Check sheet for the modelled part. Datum: model origin and axes. Units: mm. Round coordinates to 2 decimals unless told otherwise and drop trailing zeros. Write each loop counter-clockwise with the first axis right and the second up, starting at its lowest first coordinate (ties: lowest second). Pieces come first, ordered by that corner, then holes.
Item 1: Material ranges on line 1 along X through (y, z) = (1.5, -235); line 2 along Z through (x, y) = (219, 1.2); line 3 along Z through (x, y) = (235, 1.9), recorded low to high.
Item 2: Depth check by flat-ended pin: pin 1 (4 mm diameter, centred on x = 57.5, z = -190, fed in from -Y); pin 2 (4.5 mm diameter, centred on x = 15, z = -235, fed in from +Y). Enter the tip coordinate at first touch or a pass-through.
Item 3: Section check B-B, the plane z = -135.5. Record the cut outline in (x, y), plus the area to 3 significant figures.
Item 4: Section check A-A, the plane x = 59. Record the cut outline in (y, z).
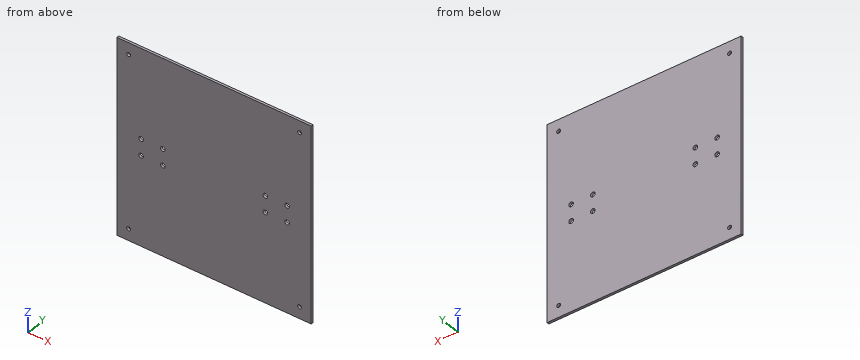
from build123d import *

# Parameters (mm, degrees)
SKETCH1_W           = 250
SKETCH1_H           = 250
BOSS_EXTRUDE1_DEPTH = 3
SKETCH2_R           = 2.5
SKETCH2_R_2         = 3
CUT_EXTRUDE1_DEPTH  = 354.566118286


with BuildPart() as part:
    # Sketch1 → Boss-Extrude1 (new body)
    with BuildSketch(Plane(origin=(0, 0, 0), x_dir=(1, 0, 0), z_dir=(0, 1, 0))):
        with Locations((125, 125)):
            Rectangle(SKETCH1_W, SKETCH1_H)
    extrude(amount=BOSS_EXTRUDE1_DEPTH)

    # Sketch2 → Cut-Extrude1 (cut, through all)
    with BuildSketch(Plane(origin=(0, 3, 0), x_dir=(1, 0, 0), z_dir=(0, 1, 0))):
        with Locations(Location((15, 235, 0), (0, 0, 270))):
            Circle(SKETCH2_R)
        with Locations(Location((235, 235, 0), (0, 0, 270))):
            Circle(SKETCH2_R)
        with Locations(Location((235, 15, 0), (0, 0, 270))):
            Circle(SKETCH2_R)
        with Locations(Location((15, 15, 0), (0, 0, 270))):
            Circle(SKETCH2_R)
        with Locations(Location((31, 135.5, 0), (0, 0, 270))):
            Circle(SKETCH2_R_2)
        with Locations(Location((59, 135.5, 0), (0, 0, 270))):
            Circle(SKETCH2_R_2)
        with Locations(Location((59, 114.5, 0), (0, 0, 270))):
            Circle(SKETCH2_R_2)
        with Locations(Location((31, 114.5, 0), (0, 0, 270))):
            Circle(SKETCH2_R_2)
        with Locations(Location((191, 135.5, 0), (0, 0, 270))):
            Circle(SKETCH2_R_2)
        with Locations(Location((219, 135.5, 0), (0, 0, 270))):
            Circle(SKETCH2_R_2)
        with Locations(Location((219, 114.5, 0), (0, 0, 270))):
            Circle(SKETCH2_R_2)
        with Locations(Location((191, 114.5, 0), (0, 0, 270))):
            Circle(SKETCH2_R_2)
    extrude(amount=-CUT_EXTRUDE1_DEPTH, mode=Mode.SUBTRACT)


solid = part.part
Values found:
1. line 1: x = 0 to 12.5, 17.5 to 232.5, 237.5 to 250
1. line 2: z = -250 to -138.5, -132.5 to -117.5, -111.5 to 0
1. line 3: z = -250 to -237.5, -232.5 to -17.5, -12.5 to 0
2. pin 1: stops at y = 0
2. pin 2: passes through
3. outline: (0, 0) - (28, 0) - (28, 3) - (0, 3) - close; (34, 0) - (56, 0) - (56, 3) - (34, 3) - close; (62, 0) - (188, 0) - (188, 3) - (62, 3) - close; (194, 0) - (216, 0) - (216, 3) - (194, 3) - close; (222, 0) - (250, 0) - (250, 3) - (222, 3) - close
3. area: 678 mm2
4. outline: (0, -250) - (3, -250) - (3, -138.5) - (0, -138.5) - close; (0, -132.5) - (3, -132.5) - (3, -117.5) - (0, -117.5) - close; (0, -111.5) - (3, -111.5) - (3, 0) - (0, 0) - close
